Input: part model. Units: mm. Frame: model coordinates. Face numbers are marked on the shaded views. Coordinates: 2 decimals unless noted, no trailing zeros. Order: outer loops, then holes, each group sorted by start corner. A loop starts at its lowest first (then second) coordinate and runs counter-clockwise, first axis right, second up. Notation, with made-up numbers: (7, 68) -> (13, 68) arc R27 ccw to (13, 87) -> close; hole circle Ø9 at (31.25, 3). An arc over 180 degrees is marked (long way). Use one line per item in the form item = value. Start each with the question number.
1) Section query B-B on x = 0. Output: boundary loops of the cut face in (y, z), then the cut area to 3 significant figures.
2) Pin query (flat end, axial travel): pin 1 (10 mm diameter, centred on y = 2.5, z = 23.5, fed in from -X); pin 2 (1 mm diameter, centred on y = 3, z = 69, fed in from -X); pin 3 (10 mm diameter, centred on y = 6.5, z = 71.5, fed in from -X); pin 4 (8 mm diameter, centred on x = -9.5, z = 51, fed in from -Y). Return the tip coordinate at first contact, or that it passes through.
3) Section query A-A on y = -7. Output: boundary loops of the cut face in (x, z), then the cut area to 3 significant figures.
4) Draft query along Y for the marked faces 1 and 2. Return one class per face: pulls with the +Y half, pulls with the -Y half, needs draft (parallel to the pull), parting line crosses it, or undercut.
5) Ray query, line 1 along Y through (x, z) = (-0.25, 84); line 2 along X through (y, z) = (0, 62); line 3 along X through (y, z) = (-6.25, 53). Return the intervals inside material, ascending.
6) Section query D-D on y = -13. Output: boundary loops of the cut face in (x, z).
7) Section query C-C on z = 38. Output: boundary loops of the cut face in (x, y), then the cut area to 3 significant figures.
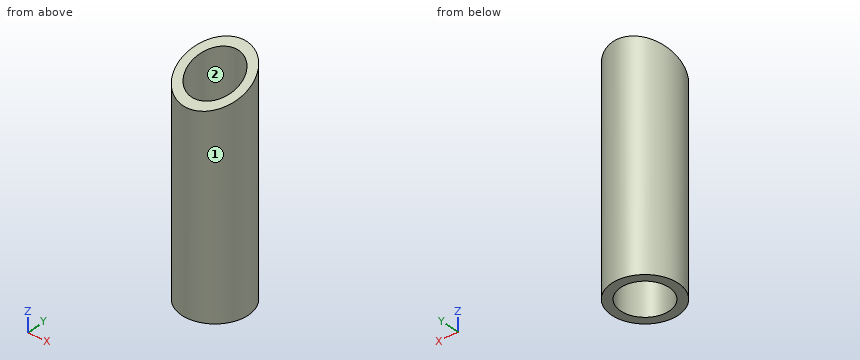
from build123d import *

# Parameters (mm, degrees)
F0_R     = 14.919644
F1_DEPTH = 101.6
F2_R     = 10.915326
F3_DEPTH = 127
F5_DEPTH = 152.4
F6_DEPTH = 152.4
F7_DEPTH = 81.026


with BuildPart() as f1:
    # F0 (on Top) → F1 (new body)
    with BuildSketch(Plane.XY):
        Circle(F0_R)
    extrude(amount=F1_DEPTH)

    # F2 (on face) → F3 (cut)
    with BuildSketch(Plane.XY.offset(101.6)):
        Circle(F2_R)
    extrude(amount=-F3_DEPTH, mode=Mode.SUBTRACT)

    # F4 (on Right) → F5 (cut)
    with BuildSketch(Plane.YZ):
        Polygon((-28.046316, 81.424184), (20.338934, 101.977214), (-28.046316, 101.977214), align=None)
    extrude(amount=-F5_DEPTH, mode=Mode.SUBTRACT)

    # F4 (on Right) → F6 (cut)
    with BuildSketch(Plane.YZ):
        Polygon((-28.046316, 81.424184), (20.338934, 101.977214), (-28.046316, 101.977214), align=None)
    extrude(amount=-F6_DEPTH, mode=Mode.SUBTRACT)

    # F4 (on Right) → F7 (cut)
    with BuildSketch(Plane.YZ):
        Polygon((-28.046316, 81.424184), (20.338934, 101.977214), (-28.046316, 101.977214), align=None)
    extrude(amount=F7_DEPTH, mode=Mode.SUBTRACT)


solid = f1.part
Answers below:
q1.outline = (-14.92, 0) -> (-10.92, 0) -> (-10.92, 88.7) -> (-14.92, 87) -> close; (10.92, 0) -> (14.92, 0) -> (14.92, 99.68) -> (10.92, 97.97) -> close
q1.area = 748 mm^2
q2.pin_1 = -14.92
q2.pin_2 = -14.71
q2.pin_3 = -14.84
q2.pin_4 = -13.87
q3.outline = (-13.18, 0) -> (-8.38, 0) -> (-8.38, 90.36) -> (-13.18, 90.36) -> close; (8.38, 0) -> (13.18, 0) -> (13.18, 90.36) -> (8.38, 90.36) -> close
q3.area = 868 mm^2
q4.face_1 = parting line crosses it
q4.face_2 = undercut
q5.line_1 = -14.92 to -10.91, 10.91 to 14.92
q5.line_2 = -14.92 to -10.92, 10.92 to 14.92
q5.line_3 = -13.55 to -8.95, 8.95 to 13.55
q6.outline = (-7.32, 0) -> (7.32, 0) -> (7.32, 87.82) -> (-7.32, 87.82) -> close
q7.outline = circle Ø29.84 at (0, 0); hole circle Ø21.83 at (0, 0)
q7.area = 325 mm^2
